Read the model definition and answer for the solid it produces. Units are mm, in the model's axes. Coordinates: 2 decimals unless noted, no trailing zeros. Loops run counter-clockwise (first coordinate to the right, second up) from the corner with the lowest first, then second, coordinate; pieces in that order, holes last. Notation, with made-up numbers: (56.5, -1) -> (76.5, -1) arc R18 ccw to (76.5, 28) -> close; hole circle Ø3 at (56, 81.25). An arc over 180 degrees is marked (long way). Answer as a JSON object with one key per item and string values. Group by question number.
1) Consider probe 1 along X at (y, z) = (1.15, 0); probe 2 along X at (y, z) = (0.65, 1.5); probe 3 along Z at (x, y) = (-0.5, 1.4). Determine where each line is inside the solid, lowest interval first. Write a range as [from, to].
2) Section C-C, the plane x = -2.5 is taken. Give the vertices of the cut face in (y, z), plus the area to 4 significant figures.
3) Section A-A, the plane z = 3 is taken. Give the vertices of the cut face in (x, y), plus the area to 3 significant figures.
4) Section B-B, the plane y = 2.2 is taken. Give the vertices of the cut face in (x, z).
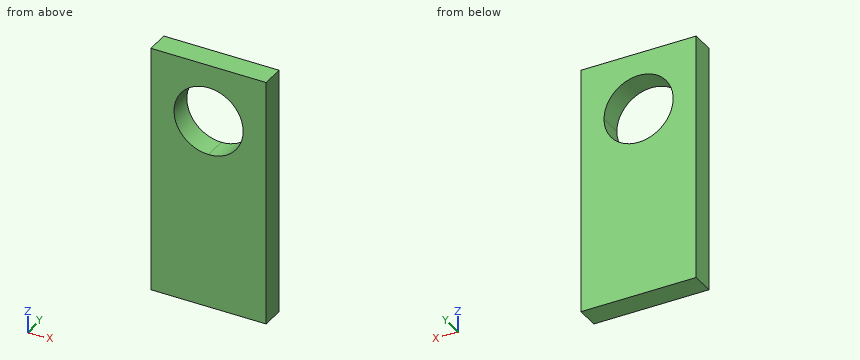
from build123d import *

# Parameters (mm, degrees)
SKETCH_1_W      = 7.5
SKETCH_1_H      = 17.5
EXTRUDE_2_DEPTH = 3


with BuildPart() as part:
    # 草图1 → 凸台-拉伸2 (new body)
    # profile 1 of 3: a face of its own
    with BuildSketch(Plane(origin=(0, 0, 0), x_dir=(1, 0, 0), z_dir=(0, 1, 0))):
        Polygon((7.5, 7.5), (0, 7.5), (-7.5, 7.5), (-7.5, -7.5), (7.5, -7.5), align=None)
        with BuildLine():
            ThreePointArc((4.5, 0), (-3.181980515, -3.181980515), (0, 4.5))
            ThreePointArc((0, 4.5), (3.181980515, 3.181980515), (4.5, 0))
        make_face(mode=Mode.SUBTRACT)
    # profile 2 of 3: a face of its own
    with BuildSketch(Plane(origin=(0, 0, 0), x_dir=(1, 0, 0), z_dir=(0, 1, 0))):
        with Locations((-3.75, 16.25)):
            Rectangle(SKETCH_1_W, SKETCH_1_H)
    # profile 3 of 3: a face of its own
    with BuildSketch(Plane(origin=(0, 0, 0), x_dir=(1, 0, 0), z_dir=(0, 1, 0))):
        with Locations((3.75, 16.25)):
            Rectangle(SKETCH_1_W, SKETCH_1_H)
    extrude(amount=EXTRUDE_2_DEPTH)


solid = part.part
Determined:
{
 "1": {"probe 1": "[-7.5, -4.5], [4.5, 7.5]", "probe 2": "[-7.5, -4.24], [4.24, 7.5]", "probe 3": "[-25, -4.47], [4.47, 7.5]"},
 "2": {"outline": "(0, -25) -> (3, -25) -> (3, -3.74) -> (0, -3.74) -> close; (0, 3.74) -> (3, 3.74) -> (3, 7.5) -> (0, 7.5) -> close", "area": "75.05 mm²"},
 "3": {"outline": "(-7.5, 0) -> (-3.35, 0) -> (-3.35, 3) -> (-7.5, 3) -> close; (3.35, 0) -> (7.5, 0) -> (7.5, 3) -> (3.35, 3) -> close", "area": "24.9 mm²"},
 "4": {"outline": "(-7.5, -25) -> (7.5, -25) -> (7.5, 7.5) -> (-7.5, 7.5) -> close; hole circle Ø9 at (0, 0)"}
}
